Autodesk Inventor part; units mm, degrees
ref_plane "YZ Plane" through (0, 0, 0) normal (1, 0, 0) x (0, 1, 0)
ref_plane "XZ Plane" through (0, 0, 0) normal (0, 1, 0) x (-1, 0, 0)
ref_plane "XY Plane" through (0, 0, 0) normal (0, 0, 1) x (1, 0, 0)
sketch "Sketch1" plane through (0, 0, 0) normal (0, 0, 1) x (1, 0, 0)
  circle A0 centre (0, 0) radius 2.8
  dimension "d0" = 5.6
extrude "Extrusion1" add sketch "Sketch1" along normal blind 1.7
fillet "Fillet3" radius 0.5 1 edges at (-2.8, 0, 0)
fillet "Fillet4" radius 1.2 1 edges at (-2.8, 0, 1.7)
sketch "Sketch2" plane through (0, 0, 1.7) normal (0, 0, 1) x (1, 0, 0)
  line L0 (-0.75, -1.299) -> (0.75, -1.299)
  line L1 (0.75, -1.299) -> (1.5, 0)
  line L2 (1.5, 0) -> (0.75, 1.299)
  line L3 (0.75, 1.299) -> (-0.75, 1.299)
  line L4 (-0.75, 1.299) -> (-1.5, 0)
  line L5 (-1.5, 0) -> (-0.75, -1.299)
  dimension "d7" = 3
extrude "Extrusion2" cut sketch "Sketch2" against normal blind 1.7
sketch "Sketch3" plane through (0, 0, 0) normal (0, 1, 0) x (-1, 0, 0)
  line L0 (0, 0) -> (1.5, 0)
  line L1 (2.3, 0) -> (-2.3, 0)
  line L2 (1.5, 0) -> (1.5, 0.8)
  line L3 (1.5, 0.8) -> (0, 0)
  line L4 (0, 0) -> (0, 2.432)
  dimension "d13" = 0
  dimension "d14" = 1.5
  dimension "d15" = 0.8
revolve "Revolution2" add sketch "Sketch3" angle 360 about axis through (0, 0, 0) along (0, 0, 1)
sketch "Sketch4" plane through (0, 0, 0) normal (0, 0, -1) x (-1, 0, 0)
  circle A0 centre (0, 0) radius 2.3
  circle A1 centre (0, 0) radius 1.5
  dimension "d18" = 3
extrude "Extrusion3" add sketch "Sketch4" along normal blind 6 contours A1
thread "Thread1"
properties part number "screw_M3_6_hex"
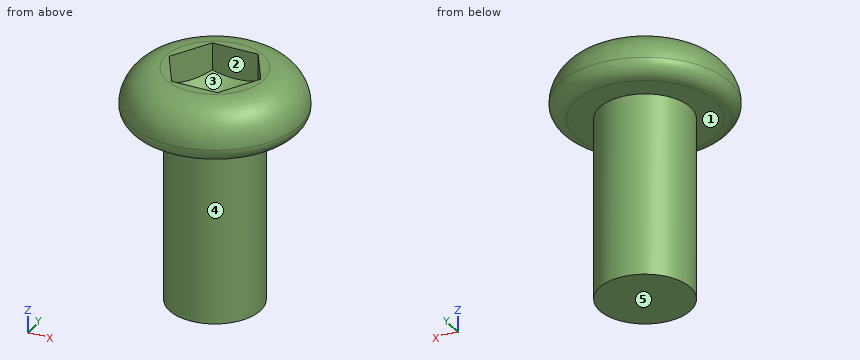
The model under review builds one solid part; all positions refer to its coordinate system, in mm. Face numbers are marked on the shaded views. A direction names the side the tool comes from. Give positions to 0.01 mm unless a question says otherwise; leave off trailing zeros. Write each loop counter-clockwise with the first axis right and the second up, starting at its lowest first coordinate (ties: lowest second). Pieces come first, ordered by that corner, then holes. Notation, with made-up numbers: M 77,54.25 L 123,54.25 A25 ccw 123,89.25 Z; hole C -4,26 d8. An arc over 180 degrees is marked long. Answer in a Markdown table with one row per item.
Item 1: Add section A-A on z = -1.5. Give the boundary of the cut face in (x, y).
Check sheet entries:
| item | result |
|---|---|
| outline | C 0,0 d3 |
Item 2: For line 1 along Y through (x, z) = (1.3, -1.25); line 2 along Z through (x, y) = (2.2, 0.5); line 3 along Y through (x, z) = (-0.1, -4.5), list the stretches that pass through material, from the lowest coordinate up.
Check sheet entries:
| item | result |
|---|---|
| line 1 | -0.75 to 0.75 |
| line 2 | 0 to 1.5 |
| line 3 | -1.5 to 1.5 |
Item 3: Tool access review of the marked faces 1 and 2: name each direction out of +Z, -Z, +X, -X, +Y, -Y from which nothing blocks a thin tool from reaching the whole face with its end or side.
Check sheet entries:
| item | result |
|---|---|
| face 1 | -Z |
| face 2 | +Z |
Item 4: Draft analysis for pull direction Y (two halves, no side actions). For the marked faces 3, 4 and 5, state which applies: +Y half, -Y half, draft (parallel to the pull), parting line (faces both ways), or undercut.
Check sheet entries:
| item | result |
|---|---|
| face 3 | undercut |
| face 4 | parting line |
| face 5 | draft |
Item 5: For P1, Ø0.5, axis at x = 0.5, z = 1, coming from the -Y side; P2, Ø3, axis at y = 1, z = -3, coming from the +X side; P3, Ø1.5, axis at x = 1, z = -1.5, coming from the -Y side, all flat-tipped, find the tip position at first contact; note any pin that passes through.
Check sheet entries:
| item | result |
|---|---|
| P1 | y = -2.74 |
| P2 | x = 1.5 |
| P3 | y = -1.48 |
